The drawing under review shows one solid part. Ordinate dimensions are in mm from its lowest x, y, z. A direction names the side the tool comes from. Round coordinates to 2 decimals unless told otherwise and drop trailing zeros. Use a Markdown table: item, result. Add a question column.
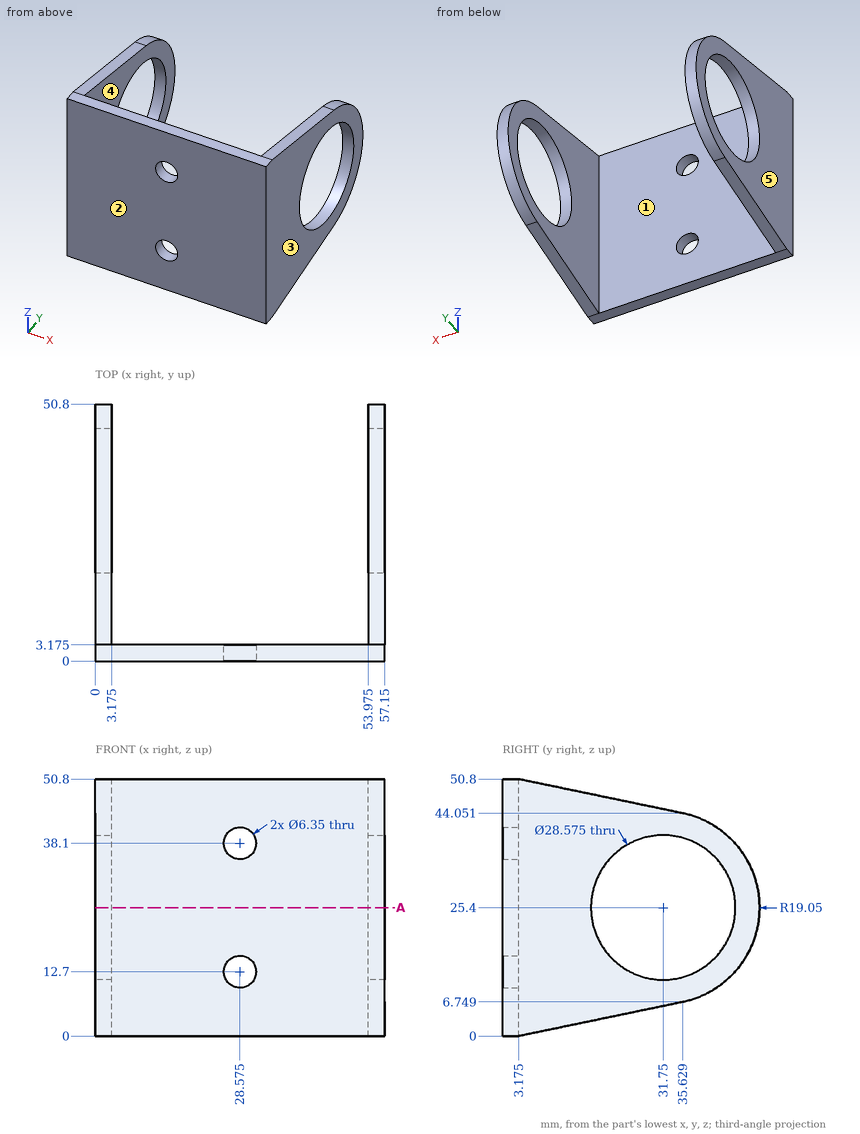
Q1. Draft analysis for pull direction X (two halves, no side actions). For the marked faces 1, 2 and 3, state which applies: released by +X, released by -X, zero draft, split by the parting line, or undercut.
Q2. To check wall thickness, follow line 1 along Y through (x, z) = (1, 25) (1 decimal); line 2 along Y through (x, z) = (41.5, 33) (1 decimal); line 3 along Z through (x, y) = (54.5, 34). State the ranges of each line that lie inside material, in increasing order.
Q3. Add section A-A, the plane z = 25.4. Give the number of separate pieces and of enclosed holes in the cut face.
Q4. For pin 1 (8 mm diameter, centred on x = 48.5, z = 29, fed in from +Y) (3 decimals), flat-tipped, find the tip position at first contact; note if it passes through.
Q5. For the marked faces 4 and 5, list the 3-axis set-ups (+Z, -Z, +X, -X, +Y, -Y) from which the entire face can be reached by the end or side of a thin tool; tool diameter is ignored.
Return value:
| question | item | result |
|---|---|---|
| 1 | face 1 | undercut |
| 1 | face 2 | zero draft |
| 1 | face 3 | released by +X |
| 2 | line 1 | 0 to 17.5, 46 to 50.8 |
| 2 | line 2 | 0 to 3.2 |
| 2 | line 3 | 6.41 to 11.29, 39.51 to 44.39 |
| 3 | separate pieces | 3 |
| 3 | enclosed holes | 0 |
| 4 | pin 1 | y = 3.175 |
| 5 | face 4 | +Z, -Z, +Y |
| 5 | face 5 | +Z, -Z, -X, +Y, -Y |
